Could you check a few things on this model? Use its own coordinates, in mm. Face numbers are marked on the shaded views. Coordinates: 2 decimals unless noted, no trailing zeros. Write each loop counter-clockwise with the first axis right and the second up, starting at its lowest first coordinate (ties: lowest second). Pieces come first, ordered by that corner, then holes. Notation, with made-up numbers: M -10,81.25 L 48,81.25 A22 cw 48,90.25 Z; hole C -21.75,40 d6. An arc over 180 degrees is marked long. Answer as CSV lines item,"result". Start each with the question number.
Item 1: We'd pull the mould along Y, two halves only. Please class the marked faces 1 and 2: +Y half, -Y half, draft (parallel to the pull), parting line (faces both ways), or undercut.
Item 2: I'm going to push flat-ended pins straight in: P1, Ø8, axis at x = 31, y = 34, coming from the -Z side; P2, Ø4, axis at x = 16, y = 60.5, coming from the +Z side (3 decimals). Where does each tip first touch, or does it pass through?
Item 3: Suppose I cut it at C-C, the plane x = -25. Write out the boundary of the cut face in (y, z) (3 decimals), and give its area (3 significant figures).
Item 4: Suppose I cut it at A-A, the plane y = 2.5. Write out the boundary of the cut face in (x, z) (3 decimals), and give its area (3 significant figures).
Item 5: If I drill on line 1 along Y through (x, z) = (-21.59, 0.2); line 2 along Y through (x, z) = (21.59, 0.3); line 3 along X through (y, z) = (-28, 0.2), over which ranges is the centre line in solid material (lowest first)? Write a range as [from, to].
Item 6: Suppose I cut it at B-B, the plane z = 0.2. Write out the boundary of the cut face in (x, y).
```python
from build123d import *

# Parameters (mm, degrees)
F0_W     = 88.9
F0_H     = 327.66
F0_R     = 12.7
F1_DEPTH = 0.5
F2_DEPTH = 0.005
F3_R     = 5.08


# Not quite as in the source:
# - a feature names something its author has since deleted; it is built from what else it names


with BuildPart() as f1:
    # F0 (on Top) → F1 (new body)
    with BuildSketch(Plane.XY):
        Rectangle(F0_W, F0_H)
        with Locations((-21.59, -139.7)):
            Circle(F0_R, mode=Mode.SUBTRACT)
        with BuildLine():
            ThreePointArc((-34.29, 139.7), (-30.5702561211, 148.6802561211), (-21.59, 152.4))
            Line((-21.59, 152.4), (4.826, 152.4))
            Line((4.826, 152.4), (4.826, 123.2959434))
            Line((4.826, 123.2959434), (34.29, 123.2959434))
            Line((34.29, 123.2959434), (34.29, -139.7))
            ThreePointArc((34.29, -139.7), (30.5702561211, -148.6802561211), (21.59, -152.4))
            Line((21.59, -152.4), (-4.826, -152.4))
            Line((-4.826, -152.4), (-4.826, -123.2959434))
            Line((-4.826, -123.2959434), (-34.29, -123.2959434))
            Line((-34.29, -123.2959434), (-34.29, 139.7))
        make_face(mode=Mode.SUBTRACT)
        with Locations((21.59, 139.7)):
            Circle(F0_R, mode=Mode.SUBTRACT)
    extrude(amount=F1_DEPTH)

    # F0 (on Top) → F2 (join)
    with BuildSketch(Plane.XY):
        with BuildLine():
            ThreePointArc((-21.59, 152.4), (-12.6097438789, 148.6802561211), (-8.89, 139.7))
            ThreePointArc((-8.89, 139.7), (-21.59, 127), (-34.29, 139.7))
            Line((-34.29, 139.7), (-34.29, -123.2959434))
            Line((-34.29, -123.2959434), (-4.826, -123.2959434))
            Line((-4.826, -123.2959434), (-4.826, -152.4))
            Line((-4.826, -152.4), (21.59, -152.4))
            ThreePointArc((21.59, -152.4), (12.6097438789, -130.7197438789), (34.29, -139.7))
            Line((34.29, -139.7), (34.29, 123.2959434))
            Line((34.29, 123.2959434), (4.826, 123.2959434))
            Line((4.826, 123.2959434), (4.826, 152.4))
            Line((4.826, 152.4), (-21.59, 152.4))
        make_face()
    extrude(amount=F2_DEPTH)

    # F3
    f3_edges = [f1.edges().sort_by_distance(p)[0] for p in [
        (-44.45, 163.83, 0.25),
        (44.45, -163.83, 0.25),
        (-44.45, -163.83, 0.25),
        (44.45, 163.83, 0.25),
        (4.826, 152.4, 0.2525),
        (4.826, 123.295943, 0.2525),
        (34.29, 123.295943, 0.2525),
        (-4.826, -152.4, 0.2525),
        (-4.826, -123.295943, 0.2525),
        (-34.29, -123.295943, 0.2525),
    ]]
    fillet(f3_edges, radius=F3_R)


solid = f1.part
```
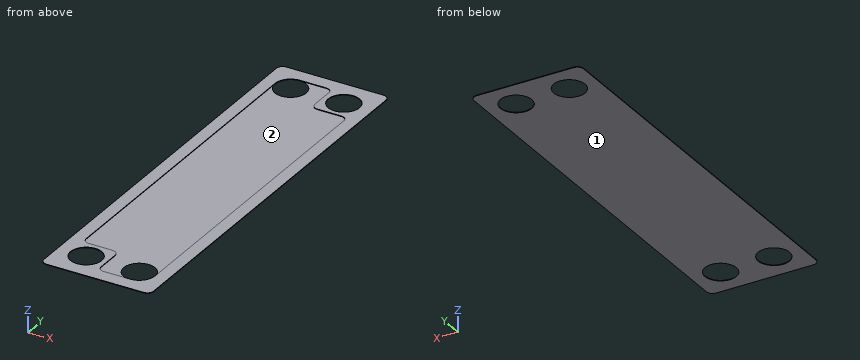
Ans:
1,face 1,"draft"
1,face 2,"undercut"
2,P1,"stops at z = 0"
2,P2,"stops at z = 0.005"
3,outline,"M -163.83,0 L -151.934,0 L -151.934,0.5 L -163.83,0.5 Z; M -127.466,0 L 127.466,0 L 127.466,0.005 L -123.296,0.005 L -123.296,0.5 L -127.466,0.5 Z; M 151.934,0 L 163.83,0 L 163.83,0.5 L 151.934,0.5 Z"
3,area,"15.2 mm^2"
4,outline,"M -44.45,0 L 44.45,0 L 44.45,0.5 L 34.29,0.5 L 34.29,0.005 L -34.29,0.005 L -34.29,0.5 L -44.45,0.5 Z"
4,area,"10.5 mm^2"
5,line 1,"y = [-163.83, -152.4], [-127, -123.3], [152.4, 163.83]"
5,line 2,"y = [-163.83, -152.4], [123.3, 127], [152.4, 163.83]"
5,line 3,"x = [-44.45, -34.29], [34.29, 44.45]"
6,outline,"M -44.45,-158.75 A5.08 ccw -39.37,-163.83 L 39.37,-163.83 A5.08 ccw 44.45,-158.75 L 44.45,158.75 A5.08 ccw 39.37,163.83 L -39.37,163.83 A5.08 ccw -44.45,158.75 Z; hole C -21.59,-139.7 d25.4; hole M -34.29,-118.22 A5.08 ccw -29.21,-123.3 L -9.91,-123.3 A5.08 cw -4.83,-128.38 L -4.83,-147.32 A5.08 ccw 0.25,-152.4 L 21.59,-152.4 A12.7 ccw 34.29,-139.7 L 34.29,118.22 A5.08 ccw 29.21,123.3 L 9.91,123.3 A5.08 cw 4.83,128.38 L 4.83,147.32 A5.08 ccw -0.25,152.4 L -21.59,152.4 A12.7 ccw -34.29,139.7 Z; hole C 21.59,139.7 d25.4"
